Source: CAD feature listing. Evaluate the final solid. Frame: model axes, mm. Face numbers are marked on the shaded views. A direction names the side the tool comes from. Coordinates: 2 decimals unless noted, no trailing zeros. Loops run counter-clockwise (first coordinate to the right, second up) from the corner with the lowest first, then second, coordinate; pieces in that order, holes last. Notation, with made-up numbers: (16.5, 63) - (37.5, 63) arc R18 ccw to (37.5, 75) - close; hole circle Ø9 at (26.5, -25). An arc over 180 degrees is marked (long way). Use CSV: the item, a comma, the result in double quotes. Start each with the question number.
```python
from build123d import *

# Parameters (mm, degrees)
SKETCH_1_W           = 50
SKETCH_1_H           = 30
EXTRUDE_1_DEPTH      = 30
SKETCH_2_W           = 10
SKETCH_2_H           = 22
SKETCH_2_W_2         = 6
SKETCH_2_H_2         = 15
CUT_EXTRUDE_1_DEPTH  = 42.833001327
SKETCH_3_W           = 5
SKETCH_3_H           = 15
EXTRUDE_2_DEPTH      = 6.5
EXTRUDE_3_DEPTH      = 6
EXTRUDE_3_DEPTH_BACK = 6


with BuildPart() as part:
    # Эскиз1 → Бобышка-Вытянуть1 (new body)
    with BuildSketch(Plane.XY):
        Rectangle(SKETCH_1_W, SKETCH_1_H)
    extrude(amount=EXTRUDE_1_DEPTH)

    # Эскиз2 → Вырез-Вытянуть1 (cut, through all)
    with BuildSketch(Plane.XY.offset(30)):
        Rectangle(SKETCH_2_W, SKETCH_2_H)
        with Locations((22, 0)):
            Rectangle(SKETCH_2_W_2, SKETCH_2_H_2)
    extrude(amount=-CUT_EXTRUDE_1_DEPTH, mode=Mode.SUBTRACT)

    # Эскиз3 → Бобышка-Вытянуть2 (add)
    with BuildSketch(Plane.XY.offset(30)):
        with Locations((-22.5, 0)):
            Rectangle(SKETCH_3_W, SKETCH_3_H)
    extrude(amount=EXTRUDE_2_DEPTH)

    # Эскиз4 → Бобышка-Вытянуть3 (add, two sides: drawn at the far end of the back side and taken through both)
    with BuildSketch(Plane(origin=(0, 0, 0), x_dir=(1, 0, 0), z_dir=(0, 1, 0)).offset(-EXTRUDE_3_DEPTH_BACK)):
        Polygon((-25, 0), (-25, 5), (-5, 0), align=None)
    extrude(amount=EXTRUDE_3_DEPTH + EXTRUDE_3_DEPTH_BACK)


solid = part.part
```
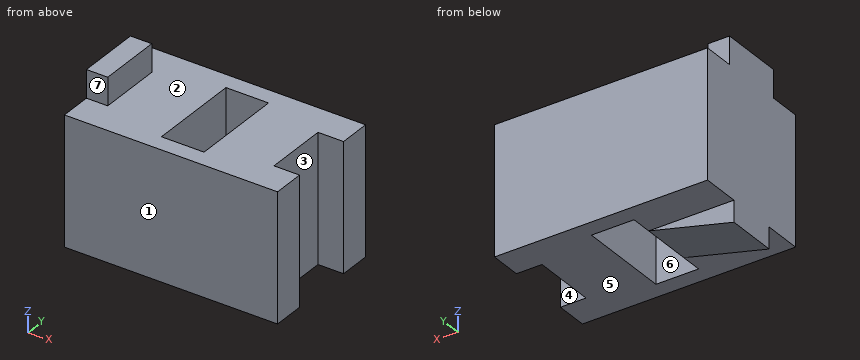
(1) Ray query, line 1 (Y direction, x = 3, z = 2); line 2 (X direction, y = -8, z = 17.5); line 3 (X direction, y = 7, z = 16.5). Return the intervals inside material, ascending. Write a range as [from, to].
(2) Section C-C on x = -19. Output: boundary loops of the cut face in (y, z), plus the area to 3 significant figures.
(3) Section D-D on y = 12.75. Output: boundary loops of the cut face in (x, z), plus the area to 3 significant figures.
(4) Reachability of the marked faces 4, 5, 6 and 7 from +Z, -Z, +X, -X, +Y, -Y: full face, straight path, thin tool, end or side. Return the list, or none.
(5) Section A-A on y = 3.25. Output: boundary loops of the cut face in (x, z), plus the area to 3 significant figures.
(6) Pin query (flat end, axial travel): pin 1 Ø2.5 at (x, z) = (-23, 34) entering from -Y; pin 2 Ø15 at (x, y) = (0, -6.5) entering from +Z; pin 3 Ø5.5 at (x, z) = (-18, -3) entering from -Y. Return the tip coordinate at first contact, or that it passes through.
(7) Section B-B on z = 6.5. Output: boundary loops of the cut face in (x, y), plus the area to 3 significant figures.
(8) Draft query along Y for the marked faces 1, 2 and 3. Return one class per face: released by +Y, released by -Y, zero draft, split by the parting line, or undercut.
Solution:
1,line 1,"y = [-15, -11], [11, 15]"
1,line 2,"x = [-25, -5], [5, 25]"
1,line 3,"x = [-25, -5], [5, 19]"
2,outline,"(-15, 0) - (-6, 0) - (-6, -3.5) - (6, -3.5) - (6, 0) - (15, 0) - (15, 30) - (-15, 30) - close"
2,area,"942 mm²"
3,outline,"(-25, 0) - (25, 0) - (25, 30) - (-25, 30) - close"
3,area,"1,500 mm²"
4,face 4,"+Z, -Z, +X"
4,face 5,"-Z, +X"
4,face 6,"+Z, -Z"
4,face 7,"+Z, +X, -X, -Y"
5,outline,"(-25, -5) - (-5, 0) - (-5, 30) - (-20, 30) - (-20, 36.5) - (-25, 36.5) - close; (5, 0) - (19, 0) - (19, 30) - (5, 30) - close"
5,area,"1,100 mm²"
6,pin 1,"stops at y = -7.5"
6,pin 2,"stops at z = 30"
6,pin 3,"stops at y = -6"
7,outline,"(-25, -15) - (25, -15) - (25, -7.5) - (19, -7.5) - (19, 7.5) - (25, 7.5) - (25, 15) - (-25, 15) - close; hole (-5, -11) - (5, -11) - (5, 11) - (-5, 11) - close"
7,area,"1,190 mm²"
8,face 1,"released by -Y"
8,face 2,"zero draft"
8,face 3,"undercut"
